The model under review builds one solid part; all positions refer to its coordinate system, in mm. Give positions to 0.01 mm unless a question says otherwise; leave off trailing zeros. Loops run counter-clockwise (first coordinate to the right, second up) from the corner with the lowest first, then second, coordinate; pieces in that order, holes last. Notation, with made-up numbers: M 11.25,40 L 29.25,40 A30 cw 29.25,62 Z; hole C 65,-5 d11. An arc over 180 degrees is marked long. Return JSON: item names as keys, results as strings.
Autodesk Inventor part; units mm, degrees
ref_plane "YZ Plane" through (0, 0, 0) normal (1, 0, 0) x (0, 1, 0)
ref_plane "XZ Plane" through (0, 0, 0) normal (0, 1, 0) x (-1, 0, 0)
ref_plane "XY Plane" through (0, 0, 0) normal (0, 0, 1) x (1, 0, 0)
sketch "スケッチ1" plane through (0, 0, 0) normal (0, 0, 1) x (1, 0, 0)
  line L0 (-100, 74.5) -> (100, 74.5)
  line L1 (100, 74.5) -> (100, -74.5)
  line L2 (100, -74.5) -> (-100, -74.5)
  line L3 (-100, -74.5) -> (-100, 74.5)
  line L4 (-100, 74.5) -> (100, -74.5) construction
  line L5 (100, 74.5) -> (-100, -74.5) construction
  circle A0 centre (0, -25.5) radius 13
  point P0 (0, 0)
  point P1 (13, -25.5)
  point P2 (-6.5, -14.2417)
  point P3 (-6.5, -36.7583)
  dimension "d4" = 26
  dimension "d0" = 200
  dimension "d1" = 149
  dimension "d10" = 360
  dimension "d19" = 100
  dimension "d20" = 49
  dimension "d22" = 0
extrude "押し出し1" add sketch "スケッチ1" against normal blind 4 contours L0 L1 L2 L3 | A0
hole "穴1" at (13, -25.5, 0) at (-6.5, -14.2417, 0) at (-6.5, -36.7583, 0) direction (0, 0, -1) diameter 5.9436 depth 10.65 tip angle 118 countersink diameter 12.6 countersink angle 90
properties part number "Board" material "アルミニウム 2014-T4"
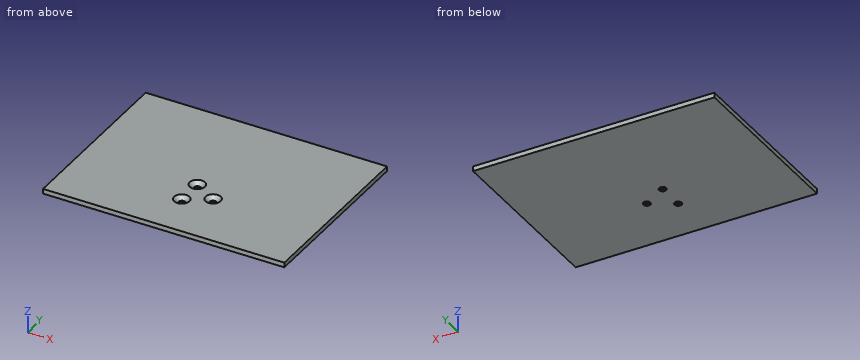
1) Consider section A-A on y = -25.5. Write out the cut boundary in (x, z).
From the geometry:
{"outline": "M -100,-4 L 10.03,-4 L 10.03,-3.33 L 6.7,0 L -100,0 Z; M 15.97,-4 L 100,-4 L 100,0 L 19.3,0 L 15.97,-3.33 Z"}
2) Wall thickness on L1, parallel to Y at x = -7, z = -3.3; L2, parallel to Y at x = 13, z = -3.65; L3, parallel to X at y = -36.5, z = -0.55: over which ranges is each line inside the solid? List them lowest first. Write a range as from..to.
From the geometry:
{"L1": "-74.5..-39.72, -33.8..-17.2, -11.28..74.5", "L2": "-74.5..-28.47, -22.53..74.5", "L3": "-100..-12.24, -0.76..100"}
3) Insertion check: pin 1 (1.5 mm diameter, centred on x = -2.5, y = 39.5, fed in from +Z). The pin has a flat end and moves straight along its axis. Give the tip position at first contact, or say it passes through.
From the geometry:
{"pin 1": "z = 0"}
4) Consider section B-B on x = -6.5. Write out the cut boundary in (y, z), then the cut area to 3 significant figures.
From the geometry:
{"outline": "M -74.5,-4 L -39.73,-4 L -39.73,-3.33 L -43.06,0 L -74.5,0 Z; M -33.79,-4 L -17.21,-4 L -17.21,-3.33 L -20.54,0 L -30.46,0 L -33.79,-3.33 Z; M -11.27,-4 L 74.5,-4 L 74.5,0 L -7.94,0 L -11.27,-3.33 Z", "area": "526 mm²"}
